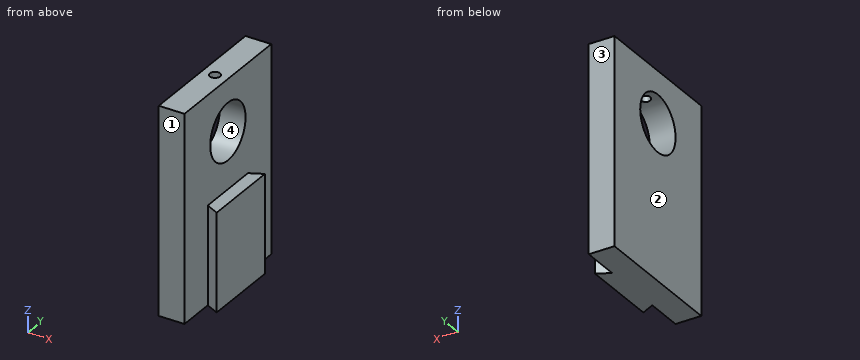
from build123d import *

# Parameters (mm, degrees)
PAD_DEPTH       = 38
SKETCH_W        = 10
SKETCH_H        = 54
PAD001_DEPTH    = 80
SKETCH002_R     = 11
POCKET_DEPTH    = 25.001
SKETCH003_R     = 2
POCKET001_DEPTH = 10


with BuildPart() as part:
    # Sketch001 → Pad (new body)
    with BuildSketch(Plane.XY):
        Polygon((-15, 0), (-15, 14.5), (-10, 12), (-10, 42), (-15, 39.5), (-15, 54), (-25, 54), (-25, 0), align=None)
    extrude(amount=PAD_DEPTH)

    # Sketch → Pad001 (join)
    with BuildSketch(Plane.XY):
        with Locations((-20, 27)):
            Rectangle(SKETCH_W, SKETCH_H)
    extrude(amount=PAD001_DEPTH)

    # Sketch002 → Pocket (cut, through all)
    with BuildSketch(Plane.YZ):
        with Locations((27, 60)):
            Circle(SKETCH002_R)
    extrude(amount=-POCKET_DEPTH, mode=Mode.SUBTRACT)

    # Sketch003 → Pocket001 (cut)
    with BuildSketch(Plane.XY.offset(80)):
        with Locations((-20, 27)):
            Circle(SKETCH003_R)
    extrude(amount=-POCKET001_DEPTH, mode=Mode.SUBTRACT)


solid = part.part
The listing builds one solid part. Answer for the finished solid, in the listing's coordinates (mm). Face numbers are marked on the shaded views. Coordinates: 2 decimals unless noted, no trailing zeros. Loops run counter-clockwise (first coordinate to the right, second up) from the corner with the lowest first, then second, coordinate; pieces in that order, holes last.
1) Find section D-D on z = 74. Write down the section's boundary in (x, y).
2) Find section C-C on x = -16. Write down the section's boundary in (y, z).
3) Flat-ended cylindrical pins translate along their axes: pin 1 Ø3 at (x, y) = (-20, 27) entering from +Z; pin 2 Ø1.5 at (x, y) = (-12.5, 23) entering from +Z. Find the tip coordinate at first contact, or state that the pin passes through.
4) Find section B-B on z = 60. Write down the section's boundary in (x, y), then the cut area to 3 significant figures.
5) Find the intervals of material crossed by L1, parallel to Z at x = -22.5, y = 27; L2, parallel to X at y = 27, z = 77.75; L3, parallel to Y at x = -20, z = 76.5, in increasing order.
6) Find section A-A on y = 27. Write down the section's boundary in (x, z), then the cut area to 3 significant figures.
7) Determine the mould class of the marked faces 1, 2, 3 and 4 for opening direction Y: pulls with the +Y half, pulls with the -Y half, needs draft (parallel to the pull), parting line crosses it, or undercut.
Values:
1. outline: (-25, 0) - (-15, 0) - (-15, 54) - (-25, 54) - close; hole circle Ø4 at (-20, 27)
2. outline: (0, 0) - (54, 0) - (54, 80) - (0, 80) - close; hole circle Ø22 at (27, 60)
3. pin 1: stops at z = 49.1
3. pin 2: stops at z = 38
4. outline: (-25, 0) - (-15, 0) - (-15, 16) - (-25, 16) - close; (-25, 38) - (-15, 38) - (-15, 54) - (-25, 54) - close
4. area: 320 mm2
5. L1: z = 0 to 49, 71 to 80
5. L2: x = -25 to -22, -18 to -15
5. L3: y = 0 to 25, 29 to 54
6. outline: (-25, 0) - (-10, 0) - (-10, 38) - (-15, 38) - (-15, 49) - (-25, 49) - close; (-25, 71) - (-22, 71) - (-22, 80) - (-25, 80) - close; (-18, 71) - (-15, 71) - (-15, 80) - (-18, 80) - close
6. area: 734 mm2
7. face 1: pulls with the -Y half
7. face 2: needs draft
7. face 3: pulls with the +Y half
7. face 4: undercut
